Geometry: see drawing. Coordinates: mm, zero at the bounding-box minimum. A direction names the side the tool comes from. Give positions to 0.01 mm unless a question says otherwise; leave off trailing zeros. Loops run counter-clockwise (first coordinate to the right, second up) from the corner with the lowest first, then second, coordinate; pieces in that order, holes last. Notation, with made-up numbers: (2.5, -6.75) -> (21.5, -6.75) arc R11 ccw to (21.5, -2.75) -> close; hole circle Ø1 at (29, -9.5). An arc over 180 degrees is marked (long way). Return JSON: item names as keys, results as strings. Group by question number.
(1) Cut plane C-C on y = 81.5. Return loops of the section in (x, z), then the cut area to 3 significant figures.
(2) Pin query (flat end, axial travel): pin 1 (4 mm diameter, centred on y = 58, z = 11, fed in from -X); pin 2 (4 mm diameter, centred on x = 12.5, y = 36, fed in from +Z); pin 3 (1.5 mm diameter, centred on y = 26.5, z = 5, fed in from +X). Return the tip coordinate at first contact, or that it passes through.
(3) Cut plane A-A on z = 7.5. Return loops of the section in (x, y), then the cut area to 3 significant figures.
(4) Access query for the marked faces 1 and 2. Directions: +Z, -Z, +X, -X, +Y, -Y. A direction counts if a zero-diameter tool reaches every point of the face in a straight line with its end or side. Return the directions, or none.
(5) Cut plane B-B on x = 7.5. Return loops of the section in (y, z).
(6) Cut plane D-D on x = 12.5. Return loops of the section in (y, z).
(7) Ray query, line 1 (Y direction, x = 2.25, z = 8); line 2 (X direction, y = 110.5, z = 7); line 3 (Y direction, x = 9, z = 10.25). Return the intervals inside material, ascending. Write a range as from..to.
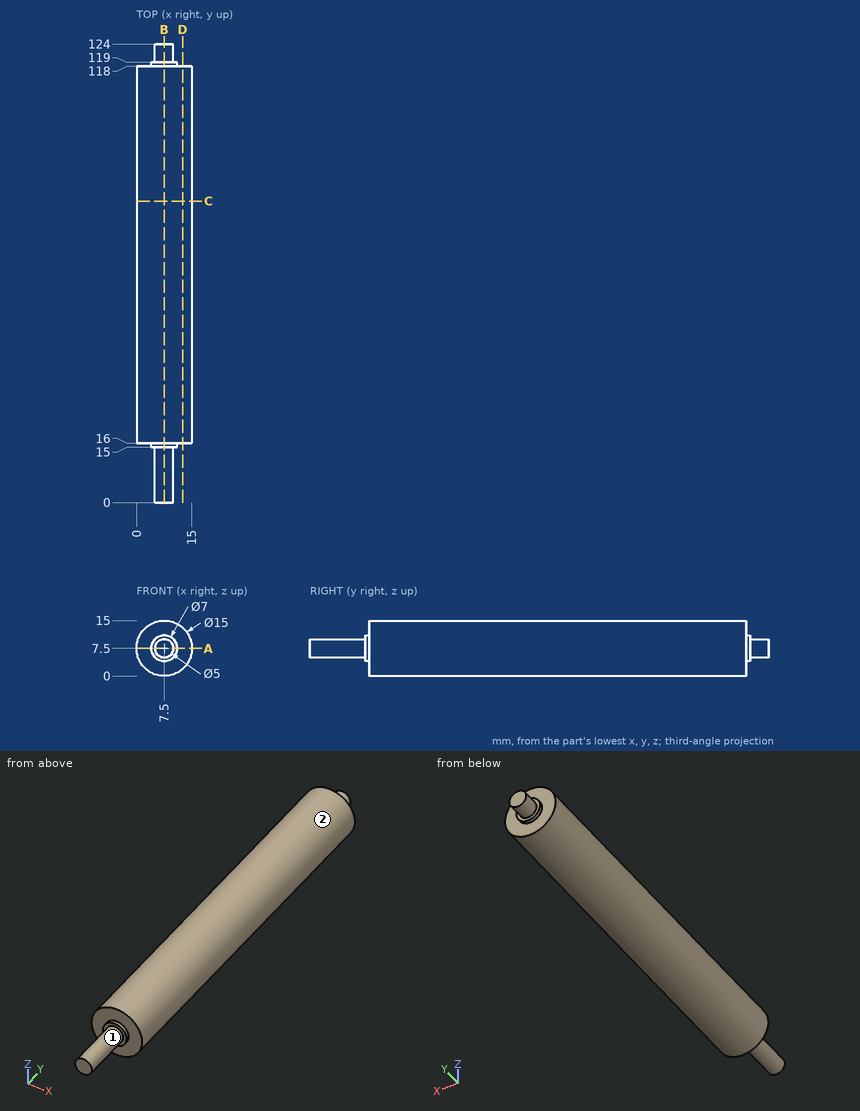
Answers:
{
 "1": {"outline": "circle Ø15 at (7.5, 7.5)", "area": "177 mm²"},
 "2": {"pin 1": "x = 0.15", "pin 2": "z = 14.37", "pin 3": "x = 14.79"},
 "3": {"outline": "(0, 16) -> (4, 16) -> (4, 15) -> (5, 15) -> (5, 0) -> (10, 0) -> (10, 15) -> (11, 15) -> (11, 16) -> (15, 16) -> (15, 118) -> (11, 118) -> (11, 119) -> (10, 119) -> (10, 124) -> (5, 124) -> (5, 119) -> (4, 119) -> (4, 118) -> (0, 118) -> close", "area": "1,640 mm²"},
 "4": {"face 1": "-Y", "face 2": "+Y, -Y"},
 "5": {"outline": "(0, 5) -> (15, 5) -> (15, 4) -> (16, 4) -> (16, 0) -> (118, 0) -> (118, 4) -> (119, 4) -> (119, 5) -> (124, 5) -> (124, 10) -> (119, 10) -> (119, 11) -> (118, 11) -> (118, 15) -> (16, 15) -> (16, 11) -> (15, 11) -> (15, 10) -> (0, 10) -> close"},
 "6": {"outline": "(16, 1.91) -> (118, 1.91) -> (118, 13.09) -> (16, 13.09) -> close"},
 "7": {"line 1": "16..118", "line 2": "0.02..14.98", "line 3": "15..119"}
}
